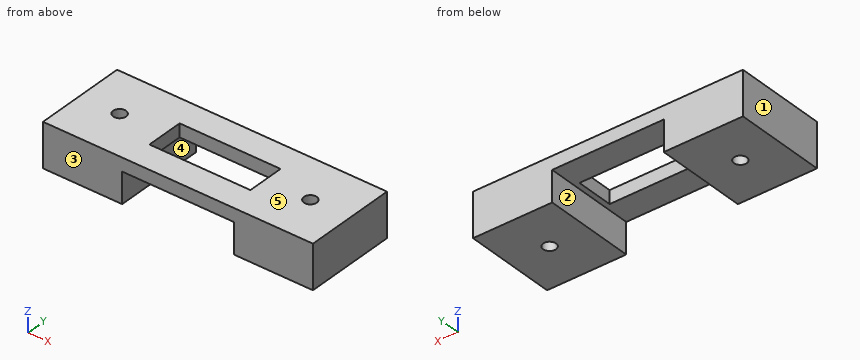
from build123d import *

# Parameters (mm, degrees)
F0_W      = 163.9416664839
F0_H      = 62.9752725363
F1_DEPTH  = 10
F2_DEPTH  = 20
F3_W      = 76.0346129537
F3_H      = 41.9552475214
F4_DEPTH  = 50
F5_DEPTH  = 10
F6_DEPTH  = 10
F7_DEPTH  = 10
F9_D      = 8.8
F11_D     = 8.8
F12_W     = 68.7855780125
F12_H     = 25.6147123873
F13_DEPTH = 25
F14_DEPTH = 10
F15_DEPTH = 10
F16_DEPTH = 5
F17_DEPTH = 5
F18_DEPTH = 15
F19_DEPTH = 5


with BuildPart() as f1:
    # F0 (on Top) → F1 (new body)
    with BuildSketch(Plane.XY):
        Rectangle(F0_W, F0_H)
    extrude(amount=F1_DEPTH)

    # F2 (add): a face of the model
    f2_faces = [f1.faces().sort_by_distance(p)[0] for p in [
        (0, 0, 10),
    ]]
    extrude(f2_faces, amount=F2_DEPTH)

    # F3 (on Front) → F4 (cut, symmetric)
    with BuildSketch(Plane.XZ):
        Rectangle(F3_W, F3_H)
    extrude(amount=F4_DEPTH, both=True, mode=Mode.SUBTRACT)

    # F5 (add): a face of the model
    f5_faces = [f1.faces().sort_by_distance(p)[0] for p in [
        (0, 0, 30),
    ]]
    extrude(f5_faces, amount=F5_DEPTH)

    # F6 (add): a face of the model
    f6_faces = [f1.faces().sort_by_distance(p)[0] for p in [
        (81.9708332419, 0, 20),
    ]]
    extrude(f6_faces, amount=F6_DEPTH)

    # F7 (add): a face of the model
    f7_faces = [f1.faces().sort_by_distance(p)[0] for p in [
        (-81.9708332419, 0, 20),
    ]]
    extrude(f7_faces, amount=F7_DEPTH)

    # F9 (through all)
    with Locations(Plane(origin=(0, 0, 0), x_dir=(1, 0, 0), z_dir=(0, 0, -1))):
        with Locations((-64.9940698594, 0)):
            Hole(F9_D / 2)

    # F11 (through all)
    with Locations(Plane(origin=(0, 0, 0), x_dir=(1, 0, 0), z_dir=(0, 0, -1))):
        with Locations((64.9940698594, 0)):
            Hole(F11_D / 2)

    # F12 (on face) → F13 (cut, symmetric)
    with BuildSketch(Plane(origin=(0, 0, 20.9776237607), x_dir=(1, 0, 0), z_dir=(0, 0, -1))):
        Rectangle(F12_W, F12_H)
    extrude(amount=F13_DEPTH, both=True, mode=Mode.SUBTRACT)

    # F14 (cut): a face of the model
    f14_faces = [f1.faces().sort_by_distance(p)[0] for p in [
        (-38.8465753115, 0, 0),
    ]]
    extrude(f14_faces, amount=-F14_DEPTH, mode=Mode.SUBTRACT)

    # F15 (cut): a face of the model
    f15_faces = [f1.faces().sort_by_distance(p)[0] for p in [
        (64.9940698594, -30.6583674335, 0),
    ]]
    extrude(f15_faces, amount=-F15_DEPTH, mode=Mode.SUBTRACT)

    # F16 (cut): a face of the model
    f16_faces = [f1.faces().sort_by_distance(p)[0] for p in [
        (64.9940698594, -30.6583674335, 10),
    ]]
    extrude(f16_faces, amount=-F16_DEPTH, mode=Mode.SUBTRACT)

    # F17 (cut): a face of the model
    f17_faces = [f1.faces().sort_by_distance(p)[0] for p in [
        (-38.8465753115, 0, 10),
    ]]
    extrude(f17_faces, amount=-F17_DEPTH, mode=Mode.SUBTRACT)

    # F18 (cut): a face of the model
    f18_faces = [f1.faces().sort_by_distance(p)[0] for p in [
        (37.0300300557, 0, 20.9776237607),
    ]]
    extrude(f18_faces, amount=-F18_DEPTH, mode=Mode.SUBTRACT)

    # F19 (add): a face of the model
    f19_faces = [f1.faces().sort_by_distance(p)[0] for p in [
        (0, 29.5434032158, 40),
    ]]
    extrude(f19_faces, amount=F19_DEPTH)


solid = f1.part
The model under review builds one solid part; all positions refer to its coordinate system, in mm. Face numbers are marked on the shaded views. A direction names the side the tool comes from. Give positions to 0.01 mm unless a question says otherwise; leave off trailing zeros. Loops run counter-clockwise (first coordinate to the right, second up) from the corner with the lowest first, then second, coordinate; pieces in that order, holes last. Notation, with made-up numbers: (56, 75) -> (78, 75) arc R16 ccw to (78, 98) -> close; hole circle Ø3 at (69, 57). An arc over 180 degrees is marked (long way). Put each result on its own line as item: value. Start each with the question number.
1. Mouldability with a two-part tool opening along X and no side actions: class the marked faces 1, 2 and 3 as released by +X, released by -X, zero draft, split by the parting line, or undercut.
2. Wall thickness on probe 1 along X at (y, z) = (0.5, 27.25); probe 2 along X at (y, z) = (-14.5, 24.5); probe 3 along Y at (x, z) = (-22, 42.75): over which ranges is each line inside the solid? List them lowest first.
3. We need section A-A on z = 33.25. State the section outline as (x, y) points.
4. For the marked faces 4 and 5, list the 3-axis set-ups (+Z, -Z, +X, -X, +Y, -Y) from which the entire face can be reached by the end or side of a thin tool; tool diameter is ignored.
5. We need section C-C on y = -9.5. State the section outline as (x, z) points, then the cut area to 3 significant figures.
6. We need section D-D on y = 0. State the section outline as (x, z) points.
7. We need section B-B on x = -22. State the section outline as (y, z) points, then the cut area to 3 significant figures.
8. Clearance check with a flat-ended pin moving along its axis: P1, Ø19, axis at x = -4, y = -10, coming from the -Z side. State where the tip first meets the part, or that it passes through.
Determined:
1. face 1: released by -X
1. face 2: undercut
1. face 3: zero draft
2. probe 1: -91.97 to -69.37, -60.62 to -38.02, 38.02 to 60.62, 69.37 to 91.97
2. probe 2: -91.97 to -38.02, 38.02 to 91.97
2. probe 3: -31.49 to -12.81, 12.81 to 31.49
3. outline: (-91.97, -31.49) -> (-38.02, -31.49) -> (-38.02, 31.49) -> (-91.97, 31.49) -> close; (38.02, -31.49) -> (91.97, -31.49) -> (91.97, 31.49) -> (38.02, 31.49) -> close; hole circle Ø8.8 at (-64.99, 0); hole circle Ø8.8 at (64.99, 0)
4. face 4: -Z, +Y, -Y
4. face 5: +Z, +X, -X, +Y, -Y
5. outline: (-91.97, 15) -> (-38.02, 15) -> (-38.02, 35.98) -> (-34.39, 35.98) -> (-34.39, 45) -> (-91.97, 45) -> close; (34.39, 35.98) -> (38.02, 35.98) -> (38.02, 15) -> (91.97, 15) -> (91.97, 45) -> (34.39, 45) -> close
5. area: 3,300 mm^2
6. outline: (-91.97, 15) -> (-69.39, 15) -> (-69.39, 45) -> (-91.97, 45) -> close; (-60.59, 15) -> (-38.02, 15) -> (-38.02, 35.98) -> (-34.39, 35.98) -> (-34.39, 45) -> (-60.59, 45) -> close; (34.39, 35.98) -> (38.02, 35.98) -> (38.02, 15) -> (60.59, 15) -> (60.59, 45) -> (34.39, 45) -> close; (69.39, 15) -> (91.97, 15) -> (91.97, 45) -> (69.39, 45) -> close
7. outline: (-31.49, 35.98) -> (-12.81, 35.98) -> (-12.81, 45) -> (-31.49, 45) -> close; (12.81, 35.98) -> (31.49, 35.98) -> (31.49, 45) -> (12.81, 45) -> close
7. area: 337 mm^2
8. P1: z = 35.98
